from build123d import *


with BuildPart() as f1:
    # F0 (on Top) → F1 (revolve)
    with BuildSketch(Plane.XY):
        with BuildLine():
            Line((0, 16.5), (0, 1.5))
            Line((0, 1.5), (2, 1.5))
            Line((2, 1.5), (2, 3.380934))
            Line((2, 3.380934), (1.538045, 3.596347))
            ThreePointArc((1.538045, 3.596347), (1.057793, 9.790565), (1.863727, 15.950878))
            Line((1.863727, 15.950878), (1.546691, 16.5))
            Line((1.546691, 16.5), (0, 16.5))
        make_face()
        with BuildLine():
            Line((-2, 1.5), (0, 1.5))
            Line((0, 1.5), (0, 16.5))
            Line((0, 16.5), (-1.546691, 16.5))
            Line((-1.546691, 16.5), (-1.863727, 15.950878))
            ThreePointArc((-1.863727, 15.950878), (-1.057793, 9.790565), (-1.538045, 3.596347))
            Line((-1.538045, 3.596347), (-2, 3.380934))
            Line((-2, 3.380934), (-2, 1.5))
        make_face()
    revolve(axis=Axis((0.653626, 0, 0), (1, 0, 0)))


solid = f1.part
CAD build for the part. Positions are in the model's coordinates, mm. Round coordinates to 2 decimals unless told otherwise and drop trailing zeros. Write each loop counter-clockwise with the first axis right and the second up, starting at its lowest first coordinate (ties: lowest second). Pieces come first, ordered by that corner, then holes.
(1) Drop flat-ended pins along their axis: P1, Ø8, axis at y = -13, z = -8, coming from the -X side; P2, Ø2, axis at x = 1.5, z = 3, coming from the -Y side; P3, Ø12, axis at y = 10.5, z = 13, coming from the +X side. Give the stop position or say it passes through.
(2) Probe line 1 along Z through (x, y) = (0.7, 0); line 2 along Z through (x, y) = (-0.2, 0.5); line 3 along Y through (x, z) = (1, 8.5). List the from-to ranges inside material, lowest first.
(3) Mould opens along Y. For faces 1 (the face through (0.03, -1.5, 0.07)), 2 (the face through (2, -1.5, -0.7)), 3 (the face through (-0.02, 15.24, -6.32)) say: pulls with the +Y half, pulls with the -Y half, needs draft (parallel to the pull), parting line crosses it, or undercut.
(4) Slice it at A-A, the plane x = 0.6. Write the cut outline in (y, z), and give its area (3 significant figures).
From the geometry:
1. P1: stops at x = -1.86
1. P2: stops at y = -16.38
1. P3: stops at x = 1.86
2. line 1: z = -16.5 to -1.5, 1.5 to 16.5
2. line 2: z = -16.49 to -1.41, 1.41 to 16.49
2. line 3: y = -14.14 to 14.14
3. face 1: undercut
3. face 2: needs draft
3. face 3: parting line crosses it
4. outline: circle Ø33 at (0, 0); hole circle Ø3 at (0, 0)
4. area: 848 mm2
